The model under review builds one solid part; all positions refer to its coordinate system, in mm. A direction names the side the tool comes from. Round coordinates to 2 decimals unless told otherwise and drop trailing zeros. Loops run counter-clockwise (first coordinate to the right, second up) from the corner with the lowest first, then second, coordinate; pieces in that order, holes last. Notation, with made-up numbers: (-25.75, 10) -> (-9.75, 10) arc R27 cw to (-9.75, 30) -> close; hole circle Ø4 at (15.5, 89). An arc over 180 degrees is marked (long way). Use a Markdown table: item, result. Add a question column.
1) Wall thickness on probe 1 along Y at (x, z) = (-6, 10); probe 2 along X at (y, z) = (-1, -15.5); probe 3 along Z at (x, y) = (-65, 93): over which ranges is each line inside the solid? List them lowest first.
2) Consider section D-D on y = 32. Give the boundary of the cut face in (x, z).
3) Insertion check: pin 1 (6 mm diameter, centred on x = 52, y = -75.5, fed in from +Z); pin 2 (8.5 mm diameter, centred on x = 75.35, y = 81.68, fed in from -Z); pin 3 (19 mm diameter, centred on x = -73.64, y = 43.89, fed in from -Z). Each pin has a flat end and moves straight along its axis. Give the tip position at first contact, or say it passes through.
4) Consider section A-A on y = 0. Give the boundary of the cut face in (x, z) (3 decimals).
5) Consider section C-C on z = -14. Give the boundary of the cut face in (x, y) (3 decimals), plus the area to 3 significant figures.
6) For faces 1 (the cylindrical face through (-70.312, 46.439, 11.448)), 2 (the cylindrical face through (-87.85, -52.15, 15.83)), 3 (the flat face through (-70, 47, 10.16)), list the 3-axis set-ups (+Z, -Z, +X, -X, +Y, -Y) from which the entire face can be reached by the end or side of a thin tool; tool diameter is ignored.
7) Consider section B-B on x = -21. Give the boundary of the cut face in (y, z).
8) Mouldability with a two-part tool opening along X and no side actions: class faces 4 (the flat face through (2, -82, 10.16)), 5 (the flat face through (0, 93, 19.05)), 6 (the cylindrical face through (-22.713, 102.283, -9.392)) as released by +X, released by -X, zero draft, split by the parting line, or undercut.
from build123d import *

# Parameters (mm, degrees)
F0_R      = 117.475
F1_DEPTH  = 12.7
F2_R      = 104.775
F3_DEPTH  = 19.05
F6_D      = 6.35
F8_D      = 8.382
F9_R      = 15.875
F9_R_2    = 4.191
F10_DEPTH = 29.21
F11_R     = 68.58
F12_DEPTH = 31.751
F13_R     = 9.525
F14_DEPTH = 6.35


with BuildPart() as f1:
    # F0 (on Top) → F1 (new body)
    with BuildSketch(Plane.XY):
        Circle(F0_R)
    extrude(amount=F1_DEPTH)

    # F2 (on face) → F3 (join)
    with BuildSketch(Plane(origin=(0, 0, 0), x_dir=(1, 0, 0), z_dir=(0, 0, -1))):
        Circle(F2_R)
    extrude(amount=F3_DEPTH)

    # F6 (through all)
    with Locations(Plane.XY.offset(12.7)):
        with Locations((-108.409797, 24.41478), (-98.740241, -50.981668), (-42.869029, -102.523227), (33.061079, -106.093029), (93.52154, -60.020723), (110.222233, 14.135946), (75.348719, 81.678248), (-67.353204, 88.387281), (5.218701, 111.002391)):
            Hole(F6_D / 2)

    # F8 (through all)
    with Locations(Plane(origin=(0, 0, -19.05), x_dir=(1, 0, 0), z_dir=(0, 0, -1))):
        with Locations((74.827591, -41.828307), (-73.638172, -43.888441), (-1.189419, 85.716748)):
            Hole(F8_D / 2)

    # F9 (on face) → F10 (cut)
    with BuildSketch(Plane(origin=(0, 0, -19.05), x_dir=(1, 0, 0), z_dir=(0, 0, -1))):
        with Locations((-73.638172, -43.888441)):
            Circle(F9_R)
        with Locations((-73.638172, -43.888441)):
            Circle(F9_R_2, mode=Mode.SUBTRACT)
        with Locations((-1.189419, 85.716748)):
            Circle(F9_R)
        with Locations((-1.189419, 85.716748)):
            Circle(F9_R_2, mode=Mode.SUBTRACT)
        with Locations((74.827591, -41.828307)):
            Circle(F9_R)
        with Locations((74.827591, -41.828307)):
            Circle(F9_R_2, mode=Mode.SUBTRACT)
    extrude(amount=-F10_DEPTH, mode=Mode.SUBTRACT)

    # F11 (on face) → F12 (cut, through all)
    with BuildSketch(Plane(origin=(0, 0, -19.05), x_dir=(1, 0, 0), z_dir=(0, 0, -1))):
        Circle(F11_R)
    extrude(amount=-F12_DEPTH, mode=Mode.SUBTRACT)

    # F13 (on face) → F14 (join)
    with BuildSketch(Plane.XY.offset(12.7)):
        with Locations((0, 92.71)):
            Circle(F13_R)
        with Locations((80.289215, -46.355)):
            Circle(F13_R)
        with Locations((-80.289215, -46.355)):
            Circle(F13_R)
    extrude(amount=F14_DEPTH)


solid = f1.part
Result set:
| question | item | result |
|---|---|---|
| 1 | probe 1 | -117.32 to -100.85, -70.59 to -68.32, 68.32 to 117.32 |
| 1 | probe 2 | -104.77 to -68.57, 68.57 to 104.77 |
| 1 | probe 3 | 0 to 12.7 |
| 2 | outline | (-113.03, 0) -> (-99.77, 0) -> (-99.77, -19.05) -> (-84.16, -19.05) -> (-84.16, 10.16) -> (-63.12, 10.16) -> (-63.12, -19.05) -> (-60.66, -19.05) -> (-60.66, 12.7) -> (-113.03, 12.7) -> close; (60.66, -19.05) -> (62.36, -19.05) -> (62.36, 10.16) -> (87.29, 10.16) -> (87.29, -19.05) -> (99.77, -19.05) -> (99.77, 0) -> (113.03, 0) -> (113.03, 12.7) -> (60.66, 12.7) -> close |
| 3 | pin 1 | z = 12.7 |
| 3 | pin 2 | z = 0 |
| 3 | pin 3 | z = 10.16 |
| 4 | outline | (-117.475, 0) -> (-104.775, 0) -> (-104.775, -19.05) -> (-68.58, -19.05) -> (-68.58, 12.7) -> (-117.475, 12.7) -> close; (68.58, -19.05) -> (104.775, -19.05) -> (104.775, 0) -> (117.475, 0) -> (117.475, 12.7) -> (68.58, 12.7) -> close |
| 5 | outline | circle Ø209.55 at (0, 0); hole circle Ø31.75 at (-73.638, 43.888); hole circle Ø137.16 at (0, 0); hole circle Ø31.75 at (-1.189, -85.717); hole circle Ø31.75 at (74.828, 41.828) |
| 5 | area | 17,300 mm2 |
| 6 | face 1 | +Z, -Z |
| 6 | face 2 | +Z |
| 6 | face 3 | -Z |
| 7 | outline | (-115.58, 0) -> (-102.65, 0) -> (-102.65, -19.05) -> (-65.29, -19.05) -> (-65.29, 12.7) -> (-115.58, 12.7) -> close; (65.29, -19.05) -> (102.65, -19.05) -> (102.65, 0) -> (115.58, 0) -> (115.58, 12.7) -> (65.29, 12.7) -> close |
| 8 | face 4 | undercut |
| 8 | face 5 | zero draft |
| 8 | face 6 | split by the parting line |
